Verification items for this drawing (mm, ordinates from the low corner). Round coordinates to 2 decimals unless told otherwise and drop trailing zeros. Write each loop counter-clockwise with the first axis right and the second up, starting at its lowest first coordinate (ties: lowest second). Pieces come first, ordered by that corner, then holes. Notation, with made-up numbers: (-20.75, -26.75) -> (15.25, -26.75) arc R29 cw to (15.25, -2.75) -> close; hole circle Ø6 at (-6.75, 19.25). An arc over 180 degrees is marked (long way). Use one line per item in the form item = value. Start each with the question number.
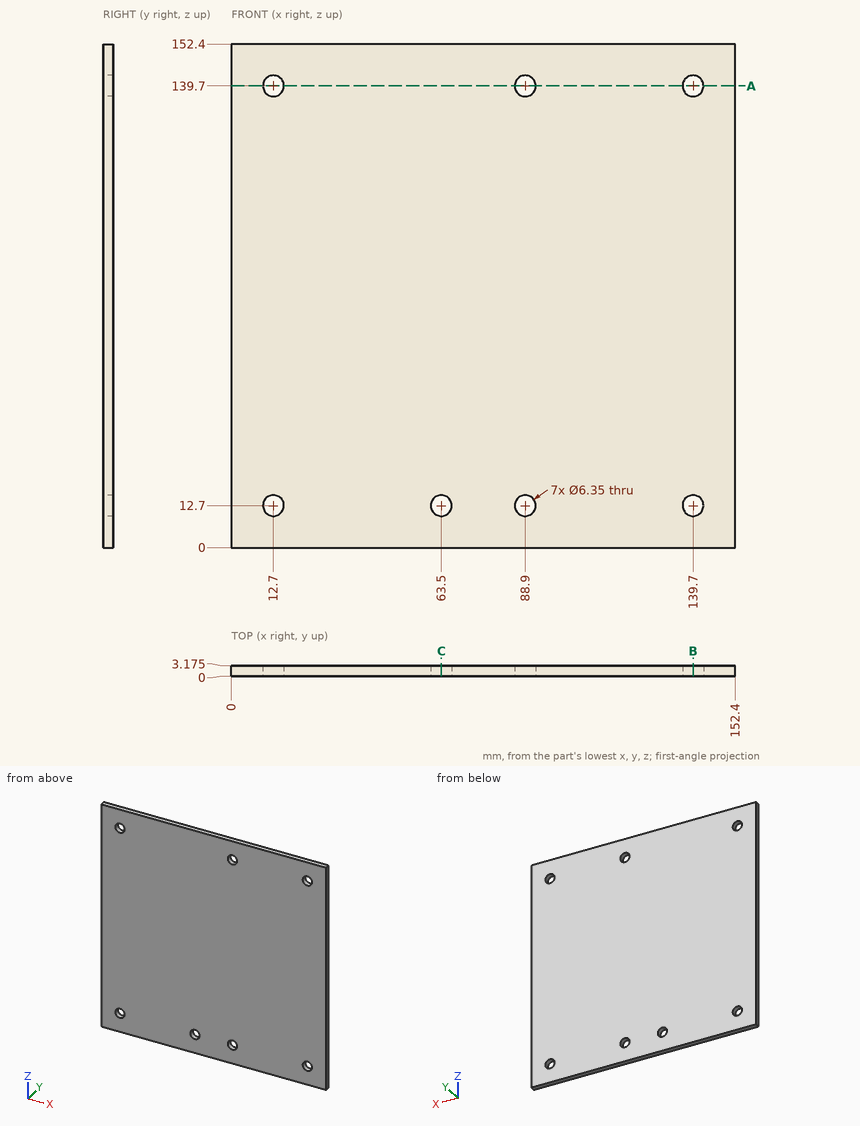
1. Depth check by flat-ended pin: pin 1 (8.5 mm diameter, centred on x = 88.9, z = 12.7, fed in from +Y) (3 decimals); pin 2 (5.5 mm diameter, centred on x = 63.5, z = 12.7, fed in from -Y). Enter the tip coordinate at first touch or a pass-through.
2. Scan lines: probe 1 along X at (y, z) = (1.7, 12.7) (3 decimals); probe 2 along X at (y, z) = (1.8, 139.7) (3 decimals); probe 3 along Z at (x, y) = (88.9, 2.1) (3 decimals). Record each from-to range of solid material in increasing order.
3. Sectioned sample at B-B (x = 139.7). Enter the section's corners in (y, z) (3 decimals).
4. Sectioned sample at C-C (x = 63.5). Enter the section's corners in (y, z) (3 decimals), and give its area (3 significant figures).
5. Sectioned sample at A-A (z = 139.7). Enter the section's corners in (x, y) (3 decimals).
Returned:
q1.pin_1 = 3.175
q1.pin_2 = through
q2.probe_1 = 0 to 9.525, 15.875 to 60.325, 66.675 to 85.725, 92.075 to 136.525, 142.875 to 152.4
q2.probe_2 = 0 to 9.525, 15.875 to 85.725, 92.075 to 136.525, 142.875 to 152.4
q2.probe_3 = 0 to 9.525, 15.875 to 136.525, 142.875 to 152.4
q3.outline = (0, 0) -> (3.175, 0) -> (3.175, 9.525) -> (0, 9.525) -> close; (0, 15.875) -> (3.175, 15.875) -> (3.175, 136.525) -> (0, 136.525) -> close; (0, 142.875) -> (3.175, 142.875) -> (3.175, 152.4) -> (0, 152.4) -> close
q4.outline = (0, 0) -> (3.175, 0) -> (3.175, 9.525) -> (0, 9.525) -> close; (0, 15.875) -> (3.175, 15.875) -> (3.175, 152.4) -> (0, 152.4) -> close
q4.area = 464 mm^2
q5.outline = (0, 0) -> (9.525, 0) -> (9.525, 3.175) -> (0, 3.175) -> close; (15.875, 0) -> (85.725, 0) -> (85.725, 3.175) -> (15.875, 3.175) -> close; (92.075, 0) -> (136.525, 0) -> (136.525, 3.175) -> (92.075, 3.175) -> close; (142.875, 0) -> (152.4, 0) -> (152.4, 3.175) -> (142.875, 3.175) -> close
